Design review of the part built by this model. Coordinates are the model's own, in mm. A direction names the side the tool comes from. Coordinates: 2 decimals unless noted, no trailing zeros. Order: outer loops, then holes, each group sorted by start corner. A loop starts at its lowest first (then second) coordinate and runs counter-clockwise, first axis right, second up. Notation, with made-up numbers: (10.25, 40.5) -> (21.25, 40.5) arc R30 ccw to (21.25, 64.5) -> close; hole circle Ø2 at (-1, 50). An arc over 180 degrees is marked (long way). Write item = value, one per line.
```python
from build123d import *

# Parameters (mm, degrees)
F2_R     = 4.7625
F3_DEPTH = 9.525
F4_DEPTH = 7.62


with BuildPart() as f1:
    # F0 (on Front) → F1 (revolve)
    with BuildSketch(Plane.XZ):
        with BuildLine():
            Line((0, 50.8), (0, 0))
            Line((0, 0), (1.5875, 0))
            add(Edge.make_bspline(
                [(1.5875, 0), (3.4055108405, 1.445712693), (8.2236413921, 5.3008235661), (23.5709920987, -0.0020492519), (30.1573484378, 8.7371555385), (31.4554715347, 12.8426796426)],
                knots=[0, 0, 0, 0, 0.271576951, 0.6434810604, 1, 1, 1, 1], degree=3))
            ThreePointArc((31.4554715347, 12.8426796426), (13.0335870575, 28.0084068393), (5.969, 50.8))
            Line((5.969, 50.8), (0, 50.8))
        make_face()
    revolve(axis=Axis((0, 0, 25.4), (0, 0, 1)))

    # F2 (on face) → F3 (cut)
    with BuildSketch(Plane.XY.offset(50.8)):
        Circle(F2_R)
    extrude(amount=-F3_DEPTH, mode=Mode.SUBTRACT)

    # F4 (cut): a face of the model
    f4_faces = [f1.faces().sort_by_distance(p)[0] for p in [
        (0, 0, 0),
    ]]
    extrude(f4_faces, amount=-F4_DEPTH, mode=Mode.SUBTRACT)


solid = f1.part
```
(1) Insertion check: pin 1 (4 mm diameter, centred on x = 1, z = 29.5, fed in from -Y); pin 2 (12 mm diameter, centred on y = 1, z = 44, fed in from -X); pin 3 (6 mm diameter, centred on y = 15.5, z = 35.5, fed in from +X) (3 decimals); pin 4 (2 mm diameter, centred on x = 18, z = 19, fed in from -Y). Each pin has a flat end and moves straight along its axis. Give the tip position at first contact, or say it passes through.
Report:
pin_1 = -13.35
pin_2 = -8.1
pin_3 = through
pin_4 = -13.86
(2) We need section B-B (z = 14.5). Write out the cut boundary in (x, y).
Report:
outline = circle Ø55.95 at (0, 0)
(3) For faces 3 (the cylindrical face through (-0.34, -1.55, 3.76)), 4 (the flat face through (0, 0, 41.275)), list the 3-axis set-ups (+Z, -Z, +X, -X, +Y, -Y) from which the entire face can be reached by the end or side of a thin tool; tool diameter is ignored.
Report:
face_3 = -Z
face_4 = +Z
(4) We need section A-A (z = 32.5). Write out the cut boundary in (x, y).
Report:
outline = circle Ø20.82 at (0, 0)
(5) For L1, parallel to Y at x = 0, z = 46; L2, parallel to Y at x = 0, z = 5; L3, parallel to Z at x = -14.5, y = -10, list the stretches that pass through material, from the lowest coordinate up.
Report:
L1 = -6.29 to -4.76, 4.76 to 6.29
L2 = -26.1 to -1.59, 1.59 to 26.1
L3 = 2.78 to 22.33
(6) The part is to be moulded in two halves that separate along Y. For faces 1 (the flat face through (-4, -3, 50.8)), 2 (the cylindrical face through (-3.78, -2.9, 46.1)), say which applies: released by +Y, released by -Y, zero draft, split by the parting line, or undercut.
Report:
face_1 = zero draft
face_2 = undercut
